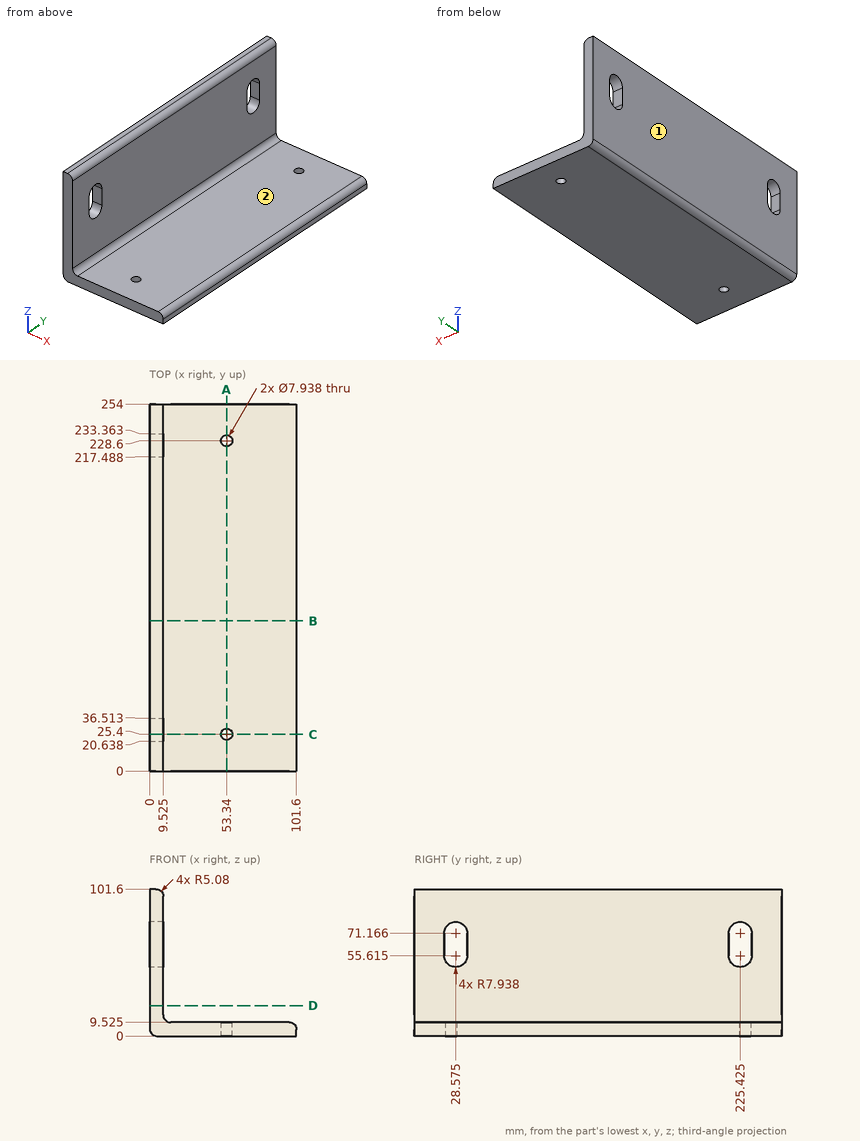
Input: dimensioned drawing with shaded views. Units: mm. Origin: part minimum x, y, z. A direction names the side the tool comes from. Give positions to 0.01 mm unless a question says otherwise; leave off trailing zeros. Order: outer loops, then holes, each group sorted by start corner. A loop starts at its lowest first (then second) coordinate and runs counter-clockwise, first axis right, second up. Notation, with made-up numbers: (-31, 45) -> (-7, 45) arc R14 ccw to (-7, 71) -> close; hole circle Ø9 at (89, -39). An arc over 180 degrees is marked (long way). Answer as a JSON object with one key per item and string values.
Q1. First-contact query: pin 1 (5 mm diameter, centred on x = 53.34, y = 25.4, fed in from -Z); pin 2 (10 mm diameter, centred on y = 164.5, z = 66, fed in from +X) (1 decimal); pin 3 (6 mm diameter, centred on x = 17, y = 26, fed in from +Z); pin 4 (10.5 mm diameter, centred on x = 53.34, y = 228.6, fed in from +Z) (1 decimal). Flat tips, straight axial feed; report the tip coordinate or a pass-through.
Entries:
{"pin 1": "passes through", "pin 2": "stops at x = 9.5", "pin 3": "stops at z = 9.56", "pin 4": "stops at z = 9.5"}
Q2. Section C-C (y = 25.4). Output: boundary loops of the cut face in (x, z) (1 decimal).
Entries:
{"outline": "(0, 5.1) arc R5.1 ccw to (5.1, 0) -> (49.4, 0) -> (49.4, 9.5) -> (14.6, 9.5) arc R5.1 cw to (9.5, 14.6) -> (9.5, 48.3) -> (0, 48.3) -> close; (0, 78.4) -> (9.5, 78.4) -> (9.5, 96.5) arc R5.1 ccw to (4.4, 101.6) -> (0, 101.6) -> close; (57.3, 0) -> (101.6, 0) -> (101.6, 4.4) arc R5.1 ccw to (96.5, 9.5) -> (57.3, 9.5) -> close"}
Q3. Material intervals for probe 1 along Y at (x, z) = (53, 7) (1 decimal); probe 2 along Z at (x, y) = (87, 219) (1 decimal); probe 3 along X at (y, z) = (228.6, 3) (1 decimal), sorted ascending.
Entries:
{"probe 1": "y = 0 to 21.4, 29.4 to 224.6, 232.6 to 254", "probe 2": "z = 0 to 9.5", "probe 3": "x = 0.4 to 49.4, 57.3 to 101.6"}
Q4. Section B-B (y = 104). Output: boundary loops of the cut face in (x, z) (1 decimal).
Entries:
{"outline": "(0, 5.1) arc R5.1 ccw to (5.1, 0) -> (101.6, 0) -> (101.6, 4.4) arc R5.1 ccw to (96.5, 9.5) -> (14.6, 9.5) arc R5.1 cw to (9.5, 14.6) -> (9.5, 96.5) arc R5.1 ccw to (4.4, 101.6) -> (0, 101.6) -> close"}
Q5. Section A-A (x = 53.34). Output: boundary loops of the cut face in (y, z) (1 decimal).
Entries:
{"outline": "(0, 0) -> (21.4, 0) -> (21.4, 9.5) -> (0, 9.5) -> close; (29.4, 0) -> (224.6, 0) -> (224.6, 9.5) -> (29.4, 9.5) -> close; (232.6, 0) -> (254, 0) -> (254, 9.5) -> (232.6, 9.5) -> close"}
Q6. Access query for the marked faces 1 and 2. Directions: +Z, -Z, +X, -X, +Y, -Y. A direction counts if a zero-diameter tool reaches every point of the face in a straight line with its end or side. Return the directions, or none.
Entries:
{"face 1": "+Z, -Z, -X, +Y, -Y", "face 2": "+Z, +X, +Y, -Y"}
Q7. Section D-D (z = 21). Output: boundary loops of the cut face in (x, y) (1 decimal).
Entries:
{"outline": "(0, 0) -> (9.5, 0) -> (9.5, 254) -> (0, 254) -> close"}
